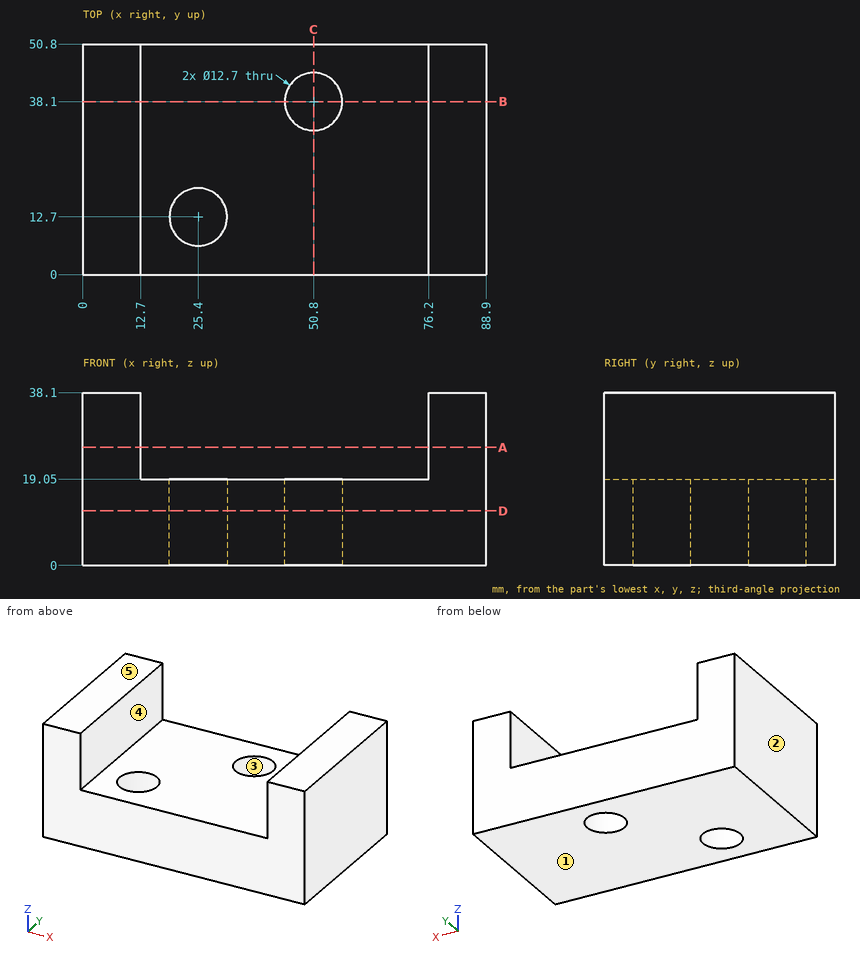
Answer from the drawing. Dimensions are ordinates in mm from the lowest x, y and z of the part. A direction names the side the tool comes from. Round coordinates to 2 decimals unless told otherwise and drop trailing zeros. Write each loop counter-clockwise with the first axis right and the second up, starting at its lowest first coordinate (ties: lowest second). Pieces come first, ordered by that corner, then holes. Notation, with made-up numbers: M 6,7 L 55,7 A32 ccw 55,37 Z; hole C -40,-28.5 d9. An arc over 180 degrees is marked long. One line per item, written item: value.
Q1. For a pull along X with two mould halves and no side action, classify the marked faces 1, 2 and 3 as +X half, -X half, draft (parallel to the pull), parting line (faces both ways), or undercut.
Data:
face 1: draft
face 2: -X half
face 3: undercut
Q2. Find section A-A on z = 26. Write down the section's boundary in (x, y), plus the area to 3 significant figures.
Data:
outline: M 0,0 L 12.7,0 L 12.7,50.8 L 0,50.8 Z; M 76.2,0 L 88.9,0 L 88.9,50.8 L 76.2,50.8 Z
area: 1,290 mm2
Q3. Find section B-B on y = 38.1. Write down the section's boundary in (x, z).
Data:
outline: M 0,0 L 44.45,0 L 44.45,19.05 L 12.7,19.05 L 12.7,38.1 L 0,38.1 Z; M 57.15,0 L 88.9,0 L 88.9,38.1 L 76.2,38.1 L 76.2,19.05 L 57.15,19.05 Z
Q4. Straight lines are drawn through the part: line 1 (X direction, y = 35.5, z = 23); line 2 (Z direction, x = 70, y = 41.5); line 3 (Y direction, x = 25.4, z = 7.5). For each, find the intervals that lie inside material, in ascending order. Write a range as [from, to].
Data:
line 1: [0, 12.7], [76.2, 88.9]
line 2: [0, 19.05]
line 3: [0, 6.35], [19.05, 50.8]
Q5. Which of the six approach directions +Z, -Z, +X, -X, +Y, -Y give full straight-line access (tool end or side, diameter ignored) to the marked faces 4 and 5?
Data:
face 4: +Z, +Y, -Y
face 5: +Z, +X, -X, +Y, -Y
Q6. Flat-ended cylindrical pins translate along their axes: pin 1 Ø9.5 at (y, z) = (20, 33) entering from -X; pin 2 Ø2 at (x, y) = (19.5, 21.5) entering from +Z. Find the tip coordinate at first contact, or state that the pin passes through.
Data:
pin 1: x = 0
pin 2: z = 19.05
Q7. Find section D-D on z = 12. Write down the section's boundary in (x, y), plus the area to 3 significant figures.
Data:
outline: M 0,0 L 88.9,0 L 88.9,50.8 L 0,50.8 Z; hole C 25.4,12.7 d12.7; hole C 50.8,38.1 d12.7
area: 4,260 mm2
Q8. Find section C-C on x = 50.8. Write down the section's boundary in (y, z), plus the area to 3 significant figures.
Data:
outline: M 0,0 L 31.75,0 L 31.75,19.05 L 0,19.05 Z; M 44.45,0 L 50.8,0 L 50.8,19.05 L 44.45,19.05 Z
area: 726 mm2
